The model under review builds one solid part; all positions refer to its coordinate system, in mm. A direction names the side the tool comes from. Coordinates: 2 decimals unless noted, no trailing zeros. Loops run counter-clockwise (first coordinate to the right, second up) from the corner with the lowest first, then second, coordinate; pieces in that order, holes last. Notation, with made-up numbers: (66, 87) -> (113, 87) arc R14 ccw to (113, 95) -> close; hole circle Ø8 at (-39, -21). An arc over 180 degrees is marked (long way). One line per question, with ' | ' between items. Start each with the question number.
from build123d import *

# Parameters (mm, degrees)
CYLINDER003_R     = 0.9
CYLINDER003_DEPTH = 10
CYLINDER004_R     = 1.175
CYLINDER004_DEPTH = 10
CYLINDER005_R     = 1.5
CYLINDER005_DEPTH = 10
CYLINDER001_R     = 1.65
CYLINDER001_DEPTH = 30
ARRAY002_X_COUNT  = 2
ARRAY002_X_PITCH  = 13
ARRAY002_Y_COUNT  = 2
ARRAY002_Y_PITCH  = 53
ARRAY_X_COUNT     = 3
ARRAY_X_PITCH     = 13
ARRAY_Y_COUNT     = 4
ARRAY_Y_PITCH     = 13
BOX_W             = 40
BOX_H             = 60
BOX_DEPTH         = 15


with BuildPart() as cylinder003:
    # Cylinder003 → Cylinder003 (new body)
    with BuildSketch(Plane(origin=(27, 17, -9), x_dir=(1, 0, 0), z_dir=(0, 0, 1))):
        Circle(CYLINDER003_R)
    extrude(amount=CYLINDER003_DEPTH)


with BuildPart() as cylinder004:
    # Cylinder004 → Cylinder004 (new body)
    with BuildSketch(Plane(origin=(27, 43, -9), x_dir=(1, 0, 0), z_dir=(0, 0, 1))):
        Circle(CYLINDER004_R)
    extrude(amount=CYLINDER004_DEPTH)


with BuildPart() as cylinder005:
    # Cylinder005 → Cylinder005 (new body)
    with BuildSketch(Plane(origin=(13, 17, -9), x_dir=(1, 0, 0), z_dir=(0, 0, 1))):
        Circle(CYLINDER005_R)
    extrude(amount=CYLINDER005_DEPTH)


with BuildPart() as hole_union:
    # Cylinder001 → Cylinder001 (new body)
    with BuildSketch(Plane.XY.offset(-20)):
        Circle(CYLINDER001_R)
    extrude(amount=CYLINDER001_DEPTH)

    # Array002 X: hole union ×2


with BuildPart() as hole_union_1:
    add(hole_union.part)
    with Locations(*[(i * ARRAY002_X_PITCH, 0, 0) for i in range(1, ARRAY002_X_COUNT)]):
        add(hole_union.part)

    # Array002 Y: hole union ×2


with BuildPart() as hole_union_2:
    add(hole_union_1.part)
    with Locations(*[(0, i * ARRAY002_Y_PITCH, 0) for i in range(1, ARRAY002_Y_COUNT)]):
        add(hole_union_1.part)


with BuildPart() as hole_union_3:
    # Array002 placement: moved
    add(hole_union_2.part.moved(Location((13.5, 3.5, 0))))

    # Fusion001: union Cylinder003, Cylinder004, Cylinder005
    add(cylinder003.part)
    add(cylinder004.part)
    add(cylinder005.part)


with BuildPart() as top_cone:
    # Cone → Cone (revolve)
    with BuildSketch(Plane(origin=(0, 0, -7), x_dir=(1, 0, 0), z_dir=(0, -1, 0))):
        Polygon((0, 0), (2.8, 0), (3, 7), (0, 7), align=None)
    revolve(axis=Axis((0, 0, -7), (0, 0, 1)))


with BuildPart() as cone_array:
    # Cone001 → Cone001 (revolve)
    with BuildSketch(Plane(origin=(0, 0, -19), x_dir=(-1, 0, 0), z_dir=(0, 1, 0))):
        Polygon((0, 0), (1.2, 0), (2.8, 12), (0, 12), align=None)
    revolve(axis=Axis((0, 0, -19), (0, 0, 1)))

    # Fusion: union top cone
    add(top_cone.part)


with BuildPart() as cone_array_1:
    # Fusion placement: moved
    add(cone_array.part.moved(Location((0, 0, 5))))

    # Array X: cone array ×3


with BuildPart() as cone_array_2:
    add(cone_array_1.part)
    with Locations(*[(i * ARRAY_X_PITCH, 0, 0) for i in range(1, ARRAY_X_COUNT)]):
        add(cone_array_1.part)

    # Array Y: cone array ×4


with BuildPart() as cone_array_3:
    add(cone_array_2.part)
    with Locations(*[(0, i * ARRAY_Y_PITCH, 0) for i in range(1, ARRAY_Y_COUNT)]):
        add(cone_array_2.part)


with BuildPart() as cone_array_4:
    # Array placement: moved
    add(cone_array_3.part.moved(Location((7, 10, 0))))


with BuildPart() as all_cut:
    # Box → Box (new body)
    with BuildSketch(Plane.XY.offset(-15)):
        with Locations((20, 30)):
            Rectangle(BOX_W, BOX_H)
    extrude(amount=BOX_DEPTH)

    # Cut: cut cone array
    add(cone_array_4.part, mode=Mode.SUBTRACT)

    # Cut001: cut hole union
    add(hole_union_3.part, mode=Mode.SUBTRACT)


solid = all_cut.part
1) Machinability: for faces 1 (the face through (40, 30, -8)), 2 (the face through (22, 25, -1)), which of the approach directions +Z, -Z, +X, -X, +Y, -Y give a long, thin tool a straight path to every point of the face, cutting with its end or side? Answer none if there is none.
2) Mouldability with a two-part tool opening along Y and no side actions: class faces 3 (the face through (20, 30, -15)), 4 (the face through (20, 0, -8)), 5 (the face through (7, 21, -8)) as +Y half, -Y half, draft (parallel to the pull), parting line (faces both ways), or undercut.
3) Wall thickness on L1, parallel to X at y = 17, z = -3.25; L2, parallel to X at y = 43, z = -2 (3 decimals); L3, parallel to X at y = 56.5, z = -11.5: over which ranges is each line inside the solid? List them lowest first.
4) Insertion check: pin 1 Ø1 at (x, z) = (16.5, -9) entering from -Y; pin 2 Ø1.6 at (x, y) = (27, 17) entering from +Z; pin 3 Ø2.5 at (x, y) = (26.5, 56.5) entering from -Z; pin 4 Ø0.7 at (x, y) = (7.5, 35.5) entering from +Z. Each pin has a flat end and moves straight along its axis. Give the tip position at first contact, or say it passes through.
5) Consider section A-A, the plane z = -3.5. Give the number of separate pieces and of enclosed holes in the cut face, plus the area to 3 significant figures.
6) Consider section C-C, the plane x = 13.5. Write out the cut boundary in (y, z).
7) Consider section B-B, the plane y = 56.5. Write out the cut boundary in (x, z), plus the area to 3 significant figures.
Filled sheet:
1) face 1: +Z, -Z, +X, +Y, -Y | face 2: +Z
2) face 3: draft | face 4: -Y half | face 5: undercut
3) L1: 0 to 11.5, 14.5 to 26.1, 27.9 to 40 | L2: 0 to 25.825, 28.175 to 40 | L3: 0 to 11.85, 15.15 to 24.85, 28.15 to 40
4) pin 1: y = 0 | pin 2: z = -9 | pin 3: through | pin 4: z = -14
5) separate pieces: 1 | enclosed holes: 19 | area: 2,100 mm^2
6) outline: (0, -15) -> (1.85, -15) -> (1.85, 0) -> (0, 0) -> close; (5.15, -15) -> (54.85, -15) -> (54.85, 0) -> (18.41, 0) -> (18.41, -9) -> (15.59, -9) -> (15.59, 0) -> (5.15, 0) -> close; (58.15, -15) -> (60, -15) -> (60, 0) -> (58.15, 0) -> close
7) outline: (0, -15) -> (11.85, -15) -> (11.85, 0) -> (0, 0) -> close; (15.15, -15) -> (24.85, -15) -> (24.85, 0) -> (15.15, 0) -> close; (28.15, -15) -> (40, -15) -> (40, 0) -> (28.15, 0) -> close | area: 501 mm^2
